The model under review builds one solid part; all positions refer to its coordinate system, in mm. Face numbers are marked on the shaded views. A direction names the side the tool comes from. Round coordinates to 2 decimals unless told otherwise and drop trailing zeros. Write each loop counter-clockwise with the first axis right and the second up, starting at its lowest first coordinate (ties: lowest second). Pieces come first, ordered by that corner, then holes. Notation, with made-up numbers: (-17, 1) - (14, 1) arc R19 cw to (14, 28) - close; hole circle Ø4 at (-36.75, -14.75). An arc over 180 degrees is marked (long way). Use one line per item in the form item = value.
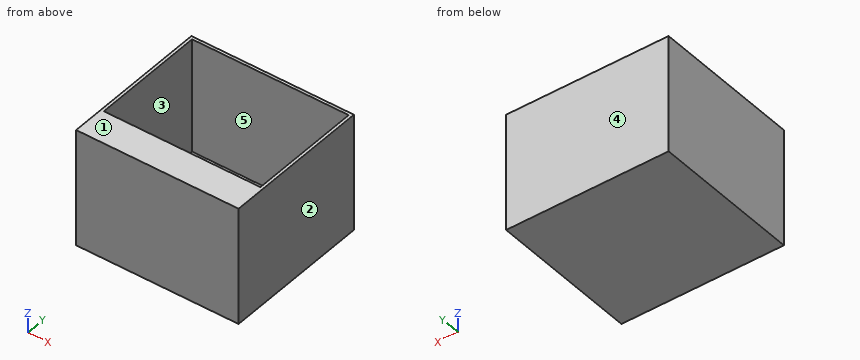
from build123d import *

# Parameters (mm, degrees)
F1_W      = 141.20084
F1_H      = 104.631812
F2_DEPTH  = 102.034964
F3_T      = -2.54
F2_FACE_W = 141.20084
F2_FACE_H = 102.034964
F4_DEPTH  = 25.4


with BuildPart() as f2:
    # F1 (on face) → F2 (new body)
    with BuildSketch(Plane.XY):
        Rectangle(F1_W, F1_H)
    extrude(amount=F2_DEPTH)

    # F3
    f3_openings = [f2.faces().sort_by_distance(p)[0] for p in [
        (0, 0, 102.034964),
    ]]
    offset(amount=F3_T, openings=f3_openings)

    # F2_face (on face) → F4 (join)
    with BuildSketch(Plane(origin=(0, -52.315906, 51.017482), x_dir=(1, 0, 0), z_dir=(0, -1, 0))):
        Rectangle(F2_FACE_W, F2_FACE_H)
    extrude(amount=F4_DEPTH)


solid = f2.part
(1) Insertion check: P1, Ø1.5, axis at x = 19, y = 23.5, coming from the +Z side. The pin has a flat end and moves straight along its axis. Give the tip position at first contact, or say it passes through.
Geometry results:
P1 = 2.54
(2) Add section B-B on x = 47.5. Write out the cut boundary in (y, z).
Geometry results:
outline = (-77.72, 0) - (52.32, 0) - (52.32, 102.03) - (49.78, 102.03) - (49.78, 2.54) - (-49.78, 2.54) - (-49.78, 102.03) - (-77.72, 102.03) - close
(3) To check wall thickness, follow L1, parallel to X at y = -0.5, z = 56; L2, parallel to Y at x = 5, z = 46; L3, parallel to Z at x = 15.5, y = 15.5. State the ranges of each line that lie inside material, in increasing order.
Geometry results:
L1 = -70.6 to -68.06, 68.06 to 70.6
L2 = -77.72 to -49.78, 49.78 to 52.32
L3 = 0 to 2.54
(4) Add section C-C on y = 33. Write out the cut boundary in (x, z).
Geometry results:
outline = (-70.6, 0) - (70.6, 0) - (70.6, 102.03) - (68.06, 102.03) - (68.06, 2.54) - (-68.06, 2.54) - (-68.06, 102.03) - (-70.6, 102.03) - close
(5) Add section A-A on z = 30. Write out the cut boundary in (x, y), then the cut area to 3 significant figures.
Geometry results:
outline = (-70.6, -77.72) - (70.6, -77.72) - (70.6, 52.32) - (-70.6, 52.32) - close; hole (-68.06, -49.78) - (68.06, -49.78) - (68.06, 49.78) - (-68.06, 49.78) - close
area = 4,810 mm2
(6) The part is to be moulded in two halves that separate along X. For the marked faces 1, 2 and 3, say which applies: +X half, -X half, draft (parallel to the pull), parting line (faces both ways), or undercut.
Geometry results:
face_1 = draft
face_2 = +X half
face_3 = undercut
(7) Machinability: for the marked faces 4 and 5, which of the approach directions +Z, -Z, +X, -X, +Y, -Y give a long, thin tool a straight path to every point of the face, cutting with its end or side? Answer none if there is none.
Geometry results:
face_4 = +Z, -Z, +X, -X, +Y
face_5 = +Z
